from build123d import *

# Parameters (mm, degrees)
BOSS_EXTRUDE1_DEPTH = 12
SKETCH3_W           = 12
SKETCH3_H           = 18
CUT_EXTRUDE1_DEPTH  = 12


with BuildPart() as part:
    # Sketch2 → Boss-Extrude1 (new body)
    with BuildSketch(Plane(origin=(0, 0, 0), x_dir=(1, 0, 0), z_dir=(0, 1, 0))):
        Polygon((0, 25), (0, 0), (142.5, 0), (142.5, 15.309556752), (352.5, 15.309556752), (352.5, 0), (495, 0), (495, 25), align=None)
    extrude(amount=BOSS_EXTRUDE1_DEPTH)

    # Sketch3 → Cut-Extrude1 (cut)
    with BuildSketch(Plane(origin=(0, 12, 0), x_dir=(1, 0, 0), z_dir=(0, 1, 0))):
        with Locations((6, 9)):
            Rectangle(SKETCH3_W, SKETCH3_H)
        with Locations((489, 9)):
            Rectangle(SKETCH3_W, SKETCH3_H)
    extrude(amount=-CUT_EXTRUDE1_DEPTH, mode=Mode.SUBTRACT)


solid = part.part
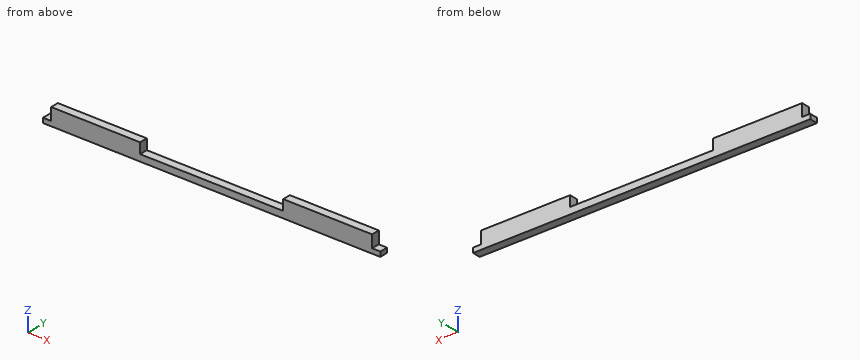
Here's how the part is built. I have some questions about the finished solid (model axes, mm). Round coordinates to 2 decimals unless told otherwise and drop trailing zeros. Write each loop counter-clockwise with the first axis right and the second up, starting at its lowest first coordinate (ties: lowest second). Pieces come first, ordered by that corner, then holes. Notation, with made-up numbers: (1, 19.25) -> (12, 19.25) arc R20 cw to (12, 27.25) -> close; hole circle Ø7 at (34, -17.75). An arc over 180 degrees is marked (long way). One line per item, written item: value.
1) Suppose I cut it at C-C on x = 161. List the corners of the cut face in (y, z) for me.
Filled sheet:
outline: (0, -25) -> (12, -25) -> (12, -15.31) -> (0, -15.31) -> close
2) If I drill on line 1 (X direction, y = 5, z = -8.25); line 2 (Z direction, x = 168.5, y = 5.25), over which ranges is the centre line in solid material (lowest first)? Write a range as [from, to].
Filled sheet:
line 1: x = [12, 142.5], [352.5, 483]
line 2: z = [-25, -15.31]
3) Suppose I cut it at B-B on y = 4.75. List the corners of the cut face in (x, z) for me, plus the area to 3 significant figures.
Filled sheet:
outline: (0, -25) -> (495, -25) -> (495, -18) -> (483, -18) -> (483, 0) -> (352.5, 0) -> (352.5, -15.31) -> (142.5, -15.31) -> (142.5, 0) -> (12, 0) -> (12, -18) -> (0, -18) -> close
area: 8,730 mm2
4) I'm going to push flat-ended pins straight in: pin 1 Ø4 at (x, y) = (337, 10) entering from +Z; pin 2 Ø4 at (y, z) = (2.5, -11) entering from +X; pin 3 Ø8 at (x, z) = (427, -16) entering from -Y; pin 4 Ø3.5 at (y, z) = (6, -10) entering from -X. Where does each tip first touch, or does it pass through?
Filled sheet:
pin 1: stops at z = -15.31
pin 2: stops at x = 483
pin 3: stops at y = 0
pin 4: stops at x = 12
5) Suppose I cut it at A-A on z = -6.5. List the corners of the cut face in (x, y) for me, plus the area to 3 significant figures.
Filled sheet:
outline: (12, 0) -> (142.5, 0) -> (142.5, 12) -> (12, 12) -> close; (352.5, 0) -> (483, 0) -> (483, 12) -> (352.5, 12) -> close
area: 3,130 mm2
